The listing builds one solid part. Answer for the finished solid, in the listing's coordinates (mm). Face numbers are marked on the shaded views. A direction names the side the tool comes from. Give positions to 0.01 mm unless a question says otherwise; leave off trailing zeros. Write each loop counter-clockwise with the first axis right and the second up, starting at its lowest first coordinate (ties: lowest second). Pieces come first, ordered by that corner, then holes. Notation, with made-up numbers: (28, 25) - (57, 25) arc R22 cw to (57, 55) - close; hole circle Ø1 at (-18.5, 48.5). An arc over 180 degrees is marked (long way). Write each question's results on one line, items separated by ' | '. Start each with the question number.
Q1. Section C-C (y = -7) is taken. Determine the outline of the cut face in (x, z) (3 decimals).
Q2. Section B-B (x = 1.75) is taken. Determine the outline of the cut face in (y, z).
Q3. For the marked faces 1, 2 and 3, determine the directions among +Z, -Z, +X, -X, +Y, -Y from which every point of the face is accessible in a straight line to the end or side of a thin tool.
Q4. Flat-ended cylindrical pins translate along their axes: pin 1 Ø5 at (y, z) = (-9, 2.5) entering from -X (3 decimals); pin 2 Ø5 at (y, z) = (-10.5, 0.5) entering from +X (3 decimals); pin 3 Ø3 at (y, z) = (-6, -2) entering from -X. Find the tip coordinate at first contact, or state that the pin passes through.
Q5. Find the intervals of material crossed by probe 1 along Y at (x, z) = (-2.75, 2.75); probe 2 along Y at (x, z) = (2, -1.25); probe 3 along Z at (x, y) = (1.5, -2.5), in increasing order.
Q6. For a pull along Z with two mould halves and no side action, classify the marked faces 4, 5 and 6 as pulls with the +Z half, pulls with the -Z half, needs draft (parallel to the pull), parting line crosses it, or undercut.
Q7. Section D-D (z = 4) is taken. Determine the outline of the cut face in (x, y).
```python
from build123d import *

# Parameters (mm, degrees)
F0_R     = 4.7625
F1_DEPTH = 6.35
F2_R     = 3.175
F3_DEPTH = 12.7
F5_DEPTH = 5.08


with BuildPart() as f1:
    # F0 (on Front) → F1 (new body)
    with BuildSketch(Plane.XZ):
        Circle(F0_R)
    extrude(amount=F1_DEPTH)

    # F2 (on face) → F3 (join)
    with BuildSketch(Plane.XZ.offset(6.35)):
        Circle(F2_R)
    extrude(amount=F3_DEPTH)

    # F4 (on face) → F5 (cut)
    with BuildSketch(Plane(origin=(0, 0, 0), x_dir=(-1, 0, 0), z_dir=(0, 1, 0))):
        Polygon((3.142612, -1.814388), (3.142612, 1.814388), (0, 3.628775), (-3.142612, 1.814388), (-3.142612, -1.814388), (0, -3.628775), align=None)
    extrude(amount=-F5_DEPTH, mode=Mode.SUBTRACT)


solid = f1.part
```
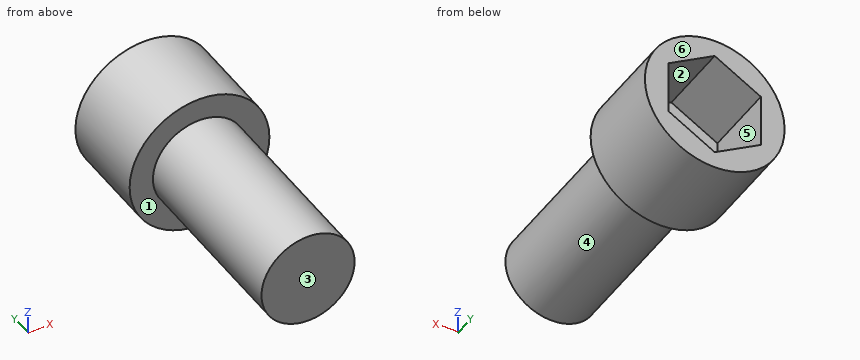
Answers below:
1) outline: circle Ø6.35 at (0, 0)
2) outline: (-19.05, -2.65) - (-6.35, -2.65) - (-6.35, -4.43) - (0, -4.43) - (0, -2.62) - (-5.08, -2.62) - (-5.08, 2.62) - (0, 2.62) - (0, 4.43) - (-6.35, 4.43) - (-6.35, 2.65) - (-19.05, 2.65) - close
3) face 1: -Y | face 2: +Y | face 3: +Z, -Z, +X, -X, -Y
4) pin 1: stops at x = -3.175 | pin 2: stops at x = 3.175 | pin 3: stops at x = -4.74
5) probe 1: y = -6.35 to 0 | probe 2: y = -19.05 to -5.08 | probe 3: z = -4.52 to -2.76, 2.76 to 4.52
6) face 4: parting line crosses it | face 5: undercut | face 6: needs draft
7) outline: (-2.58, -6.35) - (2.58, -6.35) - (2.58, 0) - (-2.58, 0) - close
